CAD build for the part. Positions are in the model's coordinates, mm. Round coordinates to 2 decimals unless told otherwise and drop trailing zeros. Write each loop counter-clockwise with the first axis right and the second up, starting at its lowest first coordinate (ties: lowest second). Pieces come first, ordered by that corner, then holes. Notation, with made-up numbers: (-36, 82.25) -> (-4, 82.25) arc R32 ccw to (-4, 117.25) -> close; hole circle Ø4 at (0.25, -13.5). An arc over 180 degrees is marked (long way). Put each result on its own line as item: value. Start each with the question number.
1. Saw through at B-B on z = -143. List the corners of the cut face in (x, y), and give its area (3 significant figures).
2. Saw through at A-A on x = 186. List the corners of the cut face in (y, z).
3. Drill centre lines: line 1 (Z direction, x = 158, y = 0.75); line 2 (Z direction, x = 152, y = 0.5); line 3 (Z direction, x = -136, y = 0.7). Where is each one in solid material? Low to high. Write a range as from..to.
from build123d import *

# Parameters (mm, degrees)
EXTRUDE1_DEPTH = 0.79375
EXTRUDE2_REACH = 2.794
SKETCH2_R      = 6.35
EXTRUDE3_REACH = 2.794
EXTRUDE4_REACH = 2.794


with BuildPart() as part:
    # Sketch1 → Extrude1 (new body)
    with BuildSketch(Plane(origin=(0, 0, 0), x_dir=(1, 0, 0), z_dir=(0, 1, 0))):
        with BuildLine():
            Line((145.25625, 434.18125), (138.034060826, 516.73125))
            Line((138.034060826, 516.73125), (-138.034060826, 516.73125))
            Line((-138.034060826, 516.73125), (-145.25625, 434.18125))
            Line((-145.25625, 434.18125), (-228.6, 434.18125))
            Line((-228.6, 434.18125), (-228.6, 199.23125))
            Line((-228.6, 199.23125), (-145.25625, 199.23125))
            ThreePointArc((-145.25625, 199.23125), (-143.670260948, 197.712995777), (-145.117890258, 196.062290917))
            Line((-145.117890258, 196.062290917), (-223.8375, 189.175217467))
            Line((-223.8375, 189.175217467), (-223.8375, 125.149782533))
            Line((-223.8375, 125.149782533), (-145.117890258, 118.262709083))
            ThreePointArc((-145.117890258, 118.262709083), (-143.668991784, 116.653544305), (-145.173166669, 115.095925614))
            Line((-145.173166669, 115.095925614), (-228.6, 110.723710546))
            Line((-228.6, 110.723710546), (-228.6, -110.723710546))
            Line((-228.6, -110.723710546), (-145.173166669, -115.095925614))
            ThreePointArc((-145.173166669, -115.095925614), (-143.668991784, -116.653544305), (-145.117890258, -118.262709083))
            Line((-145.117890258, -118.262709083), (-223.8375, -125.149782533))
            Line((-223.8375, -125.149782533), (-223.8375, -192.356281459))
            Line((-223.8375, -192.356281459), (-145.25625, -199.23125))
            Line((-145.25625, -199.23125), (145.25625, -199.23125))
            Line((145.25625, -199.23125), (223.8375, -192.356281459))
            Line((223.8375, -192.356281459), (223.8375, -125.149782533))
            Line((223.8375, -125.149782533), (145.117890258, -118.262709083))
            ThreePointArc((145.117890258, -118.262709083), (143.668991784, -116.653544305), (145.173166669, -115.095925614))
            Line((145.173166669, -115.095925614), (228.6, -110.723710546))
            Line((228.6, -110.723710546), (228.6, 110.723710546))
            Line((228.6, 110.723710546), (145.173166669, 115.095925614))
            ThreePointArc((145.173166669, 115.095925614), (143.668991784, 116.653544305), (145.117890258, 118.262709083))
            Line((145.117890258, 118.262709083), (223.8375, 125.149782533))
            Line((223.8375, 125.149782533), (223.8375, 189.175217467))
            Line((223.8375, 189.175217467), (145.117890258, 196.062290917))
            ThreePointArc((145.117890258, 196.062290917), (143.670260948, 197.712995777), (145.25625, 199.23125))
            Line((145.25625, 199.23125), (228.6, 199.23125))
            Line((228.6, 199.23125), (228.6, 434.18125))
            Line((228.6, 434.18125), (145.25625, 434.18125))
        make_face()
    extrude(amount=EXTRUDE1_DEPTH)

    # Sketch2 → Extrude2 (cut, up to next)
    with BuildSketch(Plane(origin=(0, 0.79375, 0), x_dir=(1, 0, 0), z_dir=(0, 1, 0)), mode=Mode.PRIVATE) as extrude2_sk1:
        with Locations((-145.25625, 116.68125)):
            Circle(SKETCH2_R)
    extrude2_tool1 = extrude(extrude2_sk1.sketch, amount=-EXTRUDE2_REACH, mode=Mode.PRIVATE) & part.part
    add(extrude2_tool1.solids().sort_by_distance((-145.25625, 0.79375, -116.68125))[0], mode=Mode.SUBTRACT)
    # Sketch2 → Extrude2 (cut, up to next)
    with BuildSketch(Plane(origin=(0, 0.79375, 0), x_dir=(1, 0, 0), z_dir=(0, 1, 0)), mode=Mode.PRIVATE) as extrude2_sk2:
        with Locations((-145.25625, -116.68125)):
            Circle(SKETCH2_R)
    extrude2_tool2 = extrude(extrude2_sk2.sketch, amount=-EXTRUDE2_REACH, mode=Mode.PRIVATE) & part.part
    add(extrude2_tool2.solids().sort_by_distance((-145.25625, 0.79375, 116.68125))[0], mode=Mode.SUBTRACT)
    # Sketch2 → Extrude2 (cut, up to next)
    with BuildSketch(Plane(origin=(0, 0.79375, 0), x_dir=(1, 0, 0), z_dir=(0, 1, 0)), mode=Mode.PRIVATE) as extrude2_sk3:
        with Locations((145.25625, -116.68125)):
            Circle(SKETCH2_R)
    extrude2_tool3 = extrude(extrude2_sk3.sketch, amount=-EXTRUDE2_REACH, mode=Mode.PRIVATE) & part.part
    add(extrude2_tool3.solids().sort_by_distance((145.25625, 0.79375, 116.68125))[0], mode=Mode.SUBTRACT)
    # Sketch2 → Extrude2 (cut, up to next)
    with BuildSketch(Plane(origin=(0, 0.79375, 0), x_dir=(1, 0, 0), z_dir=(0, 1, 0)), mode=Mode.PRIVATE) as extrude2_sk4:
        with Locations((145.25625, 116.68125)):
            Circle(SKETCH2_R)
    extrude2_tool4 = extrude(extrude2_sk4.sketch, amount=-EXTRUDE2_REACH, mode=Mode.PRIVATE) & part.part
    add(extrude2_tool4.solids().sort_by_distance((145.25625, 0.79375, -116.68125))[0], mode=Mode.SUBTRACT)
    # Sketch2 → Extrude2 (cut, up to next)
    with BuildSketch(Plane(origin=(0, 0.79375, 0), x_dir=(1, 0, 0), z_dir=(0, 1, 0)), mode=Mode.PRIVATE) as extrude2_sk5:
        with Locations((-145.25625, 197.64375)):
            Circle(SKETCH2_R)
    extrude2_tool5 = extrude(extrude2_sk5.sketch, amount=-EXTRUDE2_REACH, mode=Mode.PRIVATE) & part.part
    add(extrude2_tool5.solids().sort_by_distance((-145.25625, 0.79375, -197.64375))[0], mode=Mode.SUBTRACT)
    # Sketch2 → Extrude2 (cut, up to next)
    with BuildSketch(Plane(origin=(0, 0.79375, 0), x_dir=(1, 0, 0), z_dir=(0, 1, 0)), mode=Mode.PRIVATE) as extrude2_sk6:
        with Locations((145.25625, 197.64375)):
            Circle(SKETCH2_R)
    extrude2_tool6 = extrude(extrude2_sk6.sketch, amount=-EXTRUDE2_REACH, mode=Mode.PRIVATE) & part.part
    add(extrude2_tool6.solids().sort_by_distance((145.25625, 0.79375, -197.64375))[0], mode=Mode.SUBTRACT)

    # Sketch12 → Extrude3 (cut, up to next)
    with BuildSketch(Plane(origin=(0, 0.79375, 0), x_dir=(1, 0, 0), z_dir=(0, 1, 0)), mode=Mode.PRIVATE) as extrude3_sk1:
        Polygon((-138.589613839, 510.38125), (-22.225, 510.38125), (-12.7, 516.73125), (-138.034060826, 516.73125), align=None)
    extrude3_tool1 = extrude(extrude3_sk1.sketch, amount=-EXTRUDE3_REACH, mode=Mode.PRIVATE) & part.part
    add(extrude3_tool1.solids().sort_by_distance((-77.855995, 0.79375, -513.595525))[0], mode=Mode.SUBTRACT)
    # Sketch12 → Extrude3 (cut, up to next)
    with BuildSketch(Plane(origin=(0, 0.79375, 0), x_dir=(1, 0, 0), z_dir=(0, 1, 0)), mode=Mode.PRIVATE) as extrude3_sk2:
        Polygon((12.7, 516.73125), (22.225, 510.38125), (138.589613839, 510.38125), (138.034060826, 516.73125), align=None)
    extrude3_tool2 = extrude(extrude3_sk2.sketch, amount=-EXTRUDE3_REACH, mode=Mode.PRIVATE) & part.part
    add(extrude3_tool2.solids().sort_by_distance((77.855995, 0.79375, -513.595525))[0], mode=Mode.SUBTRACT)

    # Sketch13 → Extrude4 (cut, up to next)
    with BuildSketch(Plane(origin=(0, 0.79375, 0), x_dir=(1, 0, 0), z_dir=(0, 1, 0)), mode=Mode.PRIVATE) as extrude4_sk1:
        Polygon((-61.9125, -199.23125), (-55.5625, -186.53125), (-49.2125, -199.23125), align=None)
    extrude4_tool1 = extrude(extrude4_sk1.sketch, amount=-EXTRUDE4_REACH, mode=Mode.PRIVATE) & part.part
    add(extrude4_tool1.solids().sort_by_distance((-55.5625, 0.79375, 194.997917))[0], mode=Mode.SUBTRACT)
    # Sketch13 → Extrude4 (cut, up to next)
    with BuildSketch(Plane(origin=(0, 0.79375, 0), x_dir=(1, 0, 0), z_dir=(0, 1, 0)), mode=Mode.PRIVATE) as extrude4_sk2:
        Polygon((49.2125, -199.23125), (55.5625, -186.53125), (61.9125, -199.23125), align=None)
    extrude4_tool2 = extrude(extrude4_sk2.sketch, amount=-EXTRUDE4_REACH, mode=Mode.PRIVATE) & part.part
    add(extrude4_tool2.solids().sort_by_distance((55.5625, 0.79375, 194.997917))[0], mode=Mode.SUBTRACT)
    # Sketch13 → Extrude4 (cut, up to next)
    with BuildSketch(Plane(origin=(0, 0.79375, 0), x_dir=(1, 0, 0), z_dir=(0, 1, 0)), mode=Mode.PRIVATE) as extrude4_sk3:
        Polygon((-22.225, -199.23125), (-12.7, -192.88125), (12.7, -192.88125), (22.225, -199.23125), align=None)
    extrude4_tool3 = extrude(extrude4_sk3.sketch, amount=-EXTRUDE4_REACH, mode=Mode.PRIVATE) & part.part
    add(extrude4_tool3.solids().sort_by_distance((0, 0.79375, 196.344886))[0], mode=Mode.SUBTRACT)


solid = part.part
Return value:
1. outline: (-223.84, 0) -> (223.84, 0) -> (223.84, 0.79) -> (-223.84, 0.79) -> close
1. area: 355 mm^2
2. outline: (0, -434.18) -> (0.79, -434.18) -> (0.79, -199.23) -> (0, -199.23) -> close; (0, -192.49) -> (0.79, -192.49) -> (0.79, -121.84) -> (0, -121.84) -> close; (0, -112.96) -> (0.79, -112.96) -> (0.79, 112.96) -> (0, 112.96) -> close; (0, 121.84) -> (0.79, 121.84) -> (0.79, 195.67) -> (0, 195.67) -> close
3. line 1: z = -434.18..-199.23, -194.94..-119.39, -114.42..114.42, 119.39..198.12
3. line 2: z = -434.18..-199.23, -195.46..-118.86, -114.74..114.74, 118.86..198.64
3. line 3: z = -510.38..199.23
